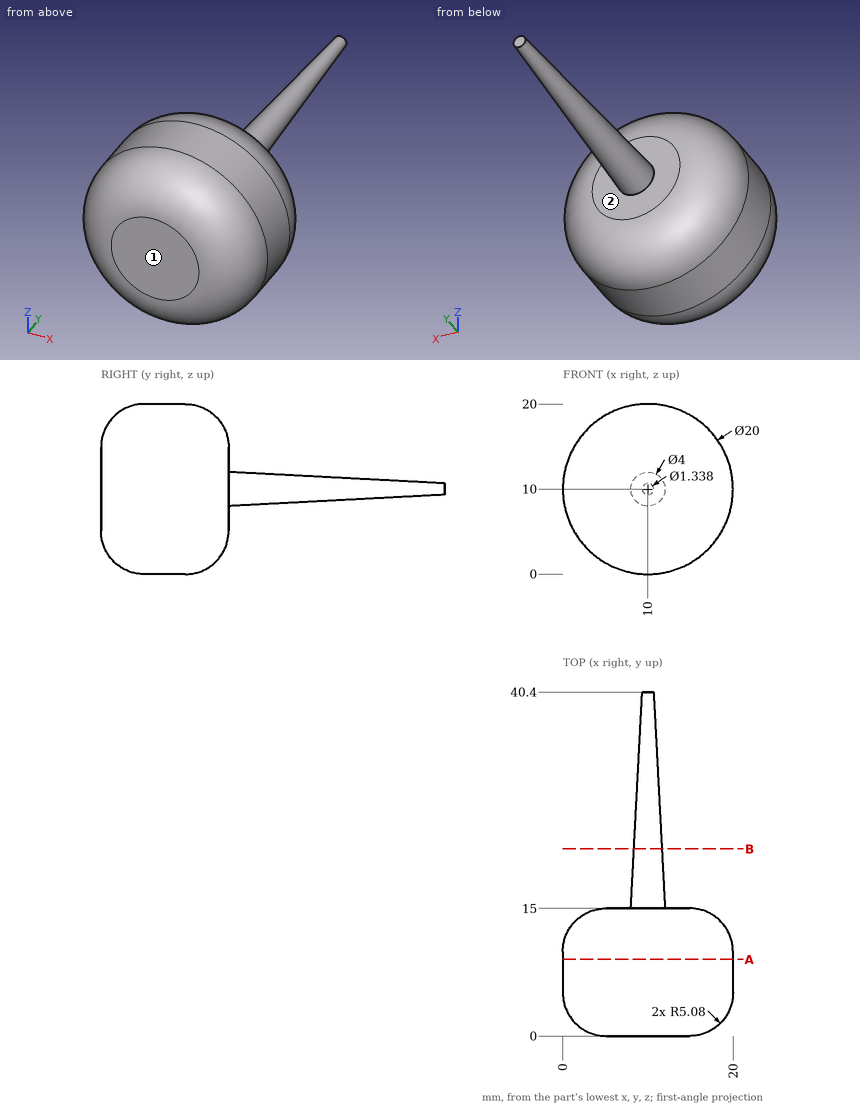
Drawing for the job (mm, zero at the part's lowest x, y, z). A direction names the side the tool comes from. Round coordinates to 2 decimals unless told otherwise and drop trailing zeros. Order: outer loops, then holes, each group sorted by start corner. A loop starts at its lowest first (then second) coordinate and runs counter-clockwise, first axis right, second up. Notation, with made-up numbers: (-38, 61.5) -> (-26, 61.5) arc R15 cw to (-26, 66.5) -> close; hole circle Ø10 at (-14, 68). An arc over 180 degrees is marked (long way). Write item = value, one per line. Start each with the question number.
(1) Cut at B-B, the plane y = 22. List the corners of the cut face in (x, z).
(2) Cut at A-A, the plane y = 9. List the corners of the cut face in (x, z).
(3) Pin check, flat tips, straight feed: P1, Ø3, axis at x = 4, y = 9.5, coming from the -Z side; P2, Ø10, axis at x = 2.5, z = 17.5, coming from the -Y side; P3, Ø1, axis at y = 13, z = 8, coming from the +X side. Stop position of each tip, or through.
(4) Probe line 1 (Y direction, x = 10.75, z = 12); line 2 (Z direction, x = 12, y = 10); line 3 (X direction, y = 10.5, z = 9.25). List the from-to ranges inside material, lowest first. Write a range as [from, to].
(5) Which spindle directions (+Z, -Z, +X, -X, +Y, -Y) get a long thin tool onto all of the face, cutting with end or side? Do the marked faces 1 and 2. Say none if no direction does.
Model answer:
q1.outline = circle Ø3.27 at (10, 10)
q2.outline = circle Ø20 at (10, 10)
q3.P1 = 1.07
q3.P2 = 0.05
q3.P3 = 19.1
q4.line_1 = [0, 15]
q4.line_2 = [0.2, 19.8]
q4.line_3 = [0.06, 19.94]
q5.face_1 = +Z, -Z, +X, -X, -Y
q5.face_2 = +Y
